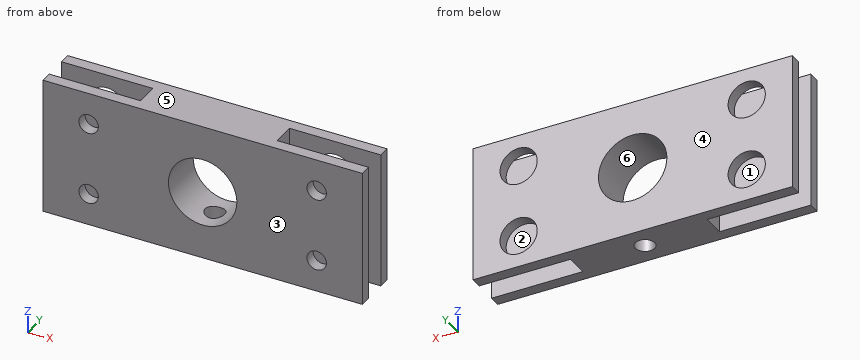
from build123d import *

# Parameters (mm, degrees)
SKETCH1_W                      = 44.45
SKETCH1_H                      = 19.05
SKETCH1_R                      = 4.7625
BOSS_EXTRUDE1_DEPTH            = 6.35
F_6_32_TAPPED_HOLE1_REACH      = 31.953
F_6_32_TAPPED_HOLE1_BORE_R     = 1.35255
SKETCH15_W                     = 12.7
SKETCH15_H                     = 3.175
CUT_EXTRUDE1_DEPTH             = 30.952890179
F_6_0_204_DIAMETER_HOLE1_D     = 5.1816
F_6_0_204_DIAMETER_HOLE1_DEPTH = 1.5875
F_6_32_TAPPED_HOLE4_D          = 2.7051


with BuildPart() as part:
    # Sketch1 → Boss-Extrude1 (new body)
    with BuildSketch(Plane(origin=(0, 0, 0), x_dir=(1, 0, 0), z_dir=(0, 1, 0))):
        Rectangle(SKETCH1_W, SKETCH1_H)
        with Locations(Location((0, 0, 0), (0, 0, 270))):
            Circle(SKETCH1_R, mode=Mode.SUBTRACT)
    extrude(amount=BOSS_EXTRUDE1_DEPTH)

    # #6-32 Tapped Hole1 bore → #6-32 Tapped Hole1 (cut, up to next)
    with BuildSketch(Plane(origin=(0, 0, -9.525), x_dir=(-1, 0, 0), z_dir=(0, 0, -1)), mode=Mode.PRIVATE) as f_6_32_tapped_hole1_sk1:
        with Locations((0, 3.175)):
            Circle(F_6_32_TAPPED_HOLE1_BORE_R)
    f_6_32_tapped_hole1_tool1 = extrude(f_6_32_tapped_hole1_sk1.sketch, amount=-F_6_32_TAPPED_HOLE1_REACH, mode=Mode.PRIVATE) & part.part
    add(f_6_32_tapped_hole1_tool1.solids().sort_by_distance((0, 3.175, -9.525))[0], mode=Mode.SUBTRACT)

    # Sketch15 → Cut-Extrude1 (cut, through all)
    with BuildSketch(Plane.XY.offset(9.525)):
        with Locations((15.875, 3.175)):
            Rectangle(SKETCH15_W, SKETCH15_H)
    cut_extrude1 = extrude(amount=-CUT_EXTRUDE1_DEPTH, mode=Mode.SUBTRACT)

    # #6 (0.204) Diameter Hole1
    with Locations(Plane(origin=(0, 6.35, 0), x_dir=(1, 0, 0), z_dir=(0, 1, 0))):
        with Locations((15.875, 5.08), (15.875, -5.08)):
            f_6_0_204_diameter_hole1 = Hole(F_6_0_204_DIAMETER_HOLE1_D / 2, depth=F_6_0_204_DIAMETER_HOLE1_DEPTH)

    # #6-32 Tapped Hole4 (through all)
    with Locations(Plane(origin=(0, 1.5875, 0), x_dir=(1, 0, 0), z_dir=(0, 1, 0))):
        with Locations((15.875, 5.08), (15.875, -5.08)):
            f_6_32_tapped_hole4 = Hole(F_6_32_TAPPED_HOLE4_D / 2)

    # Mirror3: Cut-Extrude1, #6 (0.204) Diameter Hole1, #6-32 Tapped Hole4 across plane
    add(cut_extrude1.mirror(Plane(origin=(0, 0, 0), x_dir=(0, 0, 1), z_dir=(1, 0, 0))), mode=Mode.SUBTRACT)
    add(f_6_0_204_diameter_hole1.mirror(Plane(origin=(0, 0, 0), x_dir=(0, 0, 1), z_dir=(1, 0, 0))), mode=Mode.SUBTRACT)
    add(f_6_32_tapped_hole4.mirror(Plane(origin=(0, 0, 0), x_dir=(0, 0, 1), z_dir=(1, 0, 0))), mode=Mode.SUBTRACT)


solid = part.part
Check sheet for the modelled part. Datum: model origin and axes. Units: mm. Face numbers are marked on the shaded views. A direction names the side the tool comes from. Give positions to 0.01 mm unless a question says otherwise; leave off trailing zeros. Loops run counter-clockwise (first coordinate to the right, second up) from the corner with the lowest first, then second, coordinate; pieces in that order, holes last. Notation, with made-up numbers: M -7,78 L 48,78 A20 cw 48,85 Z; hole C 6.25,45.5 d3. An arc over 180 degrees is marked long. Use a Markdown table: item, result. Add a question column.
Q1. Sectioned sample at B-B, the plane x = 0. Give the number of separate pieces and of enclosed holes in the cut face, then the cut area to 3 significant figures.
Q2. Go/stop test with a flat-tipped pin: pin 1 (4 mm diameter, centred on x = -15.875, z = -5.08, fed in from +Y). Record where the tip stops, or that it passes through.
Q3. Sectioned sample at C-C, the plane y = 4. Record the cut outline in (x, z) (1 decimal), then the cut area to 3 significant figures.
Q4. Scan lines: line 1 along Y through (x, z) = (-11.5, -3.25); line 2 along X through (y, z) = (1.25, 5.25) (3 decimals); line 3 along X through (y, z) = (5.5, -4) (3 decimals). Record each from-to range of solid material in increasing order. Write a range as [from, to].
Q5. Tool access check on the marked faces 1, 2 and 3. Record the directions out of +Z, -Z, +X, -X, +Y, -Y that give a thin tool (end or side, any length) a straight path to the whole face; none if there is none.
Q6. Mould release check, pull along Z, two halves, no side actions. Record for the marked faces 4, 5 and 6: pulls with the +Z half, pulls with the -Z half, needs draft (parallel to the pull), parting line crosses it, or undercut.
Verdict:
| question | item | result |
|---|---|---|
| 1 | separate pieces | 3 |
| 1 | enclosed holes | 0 |
| 1 | area | 47.6 mm^2 |
| 2 | pin 1 | y = 1.59 |
| 3 | outline | M -9.5,-9.5 L -1.1,-9.5 L -1.1,-4.6 A4.8 cw long 1.1,-4.6 L 1.1,-9.5 L 9.5,-9.5 L 9.5,9.5 L -9.5,9.5 Z |
| 3 | area | 281 mm^2 |
| 4 | line 1 | [0, 1.59], [4.76, 6.35] |
| 4 | line 2 | [-22.225, -17.217], [-14.533, 14.533], [17.217, 22.225] |
| 4 | line 3 | [-22.225, -18.23], [-13.52, -2.585], [2.585, 13.52], [18.23, 22.225] |
| 5 | face 1 | +Z, -Z, -X |
| 5 | face 2 | +Z, -Z, +X |
| 5 | face 3 | +Z, -Z, +X, -X, -Y |
| 6 | face 4 | needs draft |
| 6 | face 5 | pulls with the +Z half |
| 6 | face 6 | undercut |
